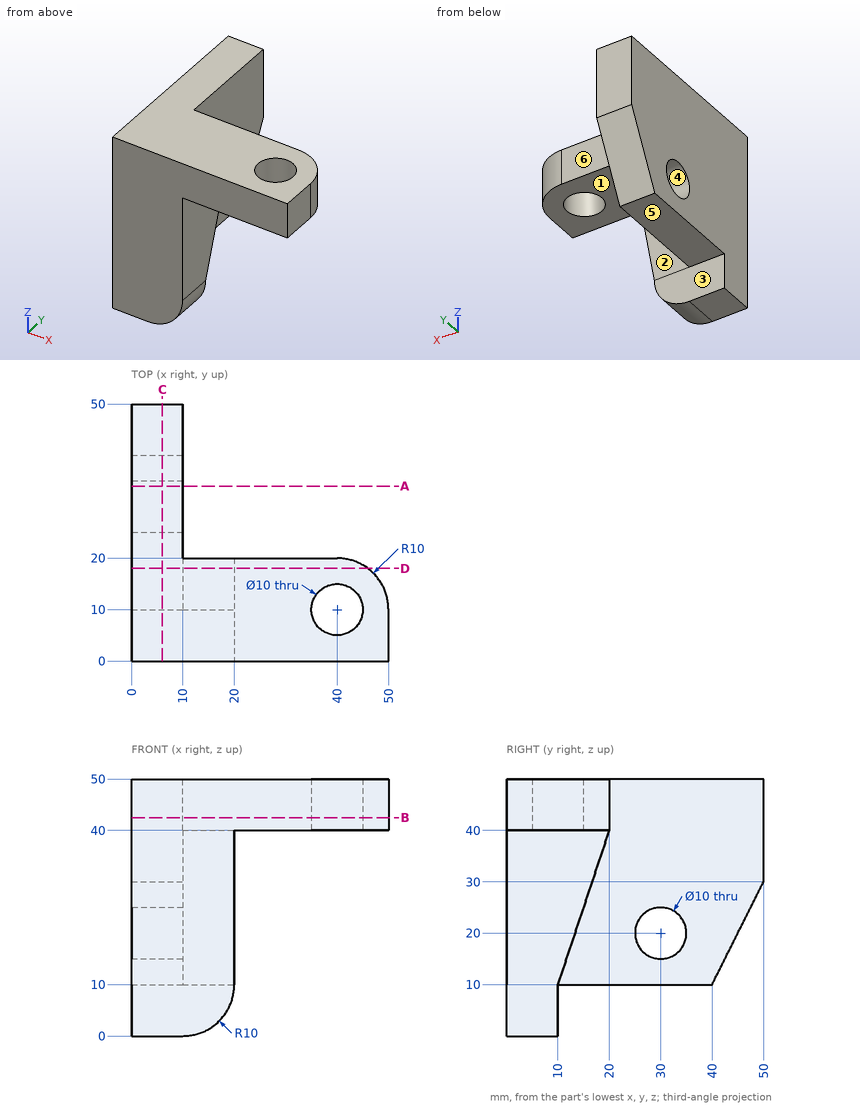
Study the drawing (mm; zero at the part's minimum x, y, z) and answer. A direction names the side the tool comes from. Give positions to 0.01 mm unless a question says otherwise; leave off trailing zeros. Loops run counter-clockwise (first coordinate to the right, second up) from the corner with the lowest first, then second, coordinate; pieces in that order, holes last. Notation, with made-up numbers: M 2.25,23.5 L 45.25,23.5 A16 ccw 45.25,42.5 Z; hole C -2.75,-20 d2. An arc over 180 degrees is marked long. One line per item, written item: value.
1. Each of these flat-tipped pins is pushed along its axis until it touches: P1, Ø22, axis at y = 14, z = 17.5, coming from the +X side; P2, Ø3, axis at y = 26, z = 12, coming from the +X side; P3, Ø16, axis at x = 35, y = 12.5, coming from the -Z side. Where does it stop, or does it pass through?
Found:
P1: x = 20
P2: x = 10
P3: z = 40
2. Section D-D on y = 18 is taken. Determine the outline of the cut face in (x, z).
Found:
outline: M 0,10 L 10,10 L 10,34 L 20,34 L 20,40 L 46,40 L 46,50 L 0,50 Z
3. Section B-B on z = 42.5 is taken. Determine the outline of the cut face in (x, y).
Found:
outline: M 0,0 L 50,0 L 50,10 A10 ccw 40,20 L 10,20 L 10,50 L 0,50 Z; hole C 40,10 d10
4. For the marked faces 1, 2 and 3, determine the directions among +Z, -Z, +X, -X, +Y, -Y from which every point of the face is accessible in a straight line to the end or side of a thin tool.
Found:
face 1: -Z, +X, +Y, -Y
face 2: -Z, +X, +Y
face 3: -Z, +X, -X, +Y
5. Section A-A on y = 34 is taken. Determine the outline of the cut face in (x, z).
Found:
outline: M 0,10 L 10,10 L 10,17 L 0,17 Z; M 0,23 L 10,23 L 10,50 L 0,50 Z
6. Find the intervals of material crossed by probe 1 along X at (y, z) = (10, 44); probe 2 along Y at (x, z) = (6, 20); probe 3 along Z at (x, y) = (3.5, 29), in increasing order.
Found:
probe 1: 0 to 35, 45 to 50
probe 2: 0 to 25, 35 to 45
probe 3: 10 to 15.1, 24.9 to 50
7. Section C-C on x = 6 is taken. Determine the outline of the cut face in (y, z), plus the area to 3 significant figures.
Found:
outline: M 0,0 L 10,0 L 10,10 L 40,10 L 50,30 L 50,50 L 0,50 Z; hole C 30,20 d10
area: 1,920 mm^2
8. For a pull along Y with two mould halves and no side action, classify the marked faces 4, 5 and 6 as pulls with the +Y half, pulls with the -Y half, needs draft (parallel to the pull), parting line crosses it, or undercut.
Found:
face 4: undercut
face 5: needs draft
face 6: pulls with the +Y half
